Design review of the part built by this model. Coordinates are the model's own, in mm. A direction names the side the tool comes from. Give positions to 0.01 mm unless a question says otherwise; leave off trailing zeros. Order: outer loops, then holes, each group sorted by start corner. A loop starts at its lowest first (then second) coordinate and runs counter-clockwise, first axis right, second up.
```python
from build123d import *

# Parameters (mm, degrees)
F0_W     = 35.8
F0_H     = 9.8
F1_DEPTH = 9.8
F2_R     = 2
F3_DEPTH = 25
F5_DEPTH = 2.4
F6_R     = 2
F7_DEPTH = 40
F8_W     = 2.4
F8_H     = 5.5
F9_DEPTH = 25


with BuildPart() as f1:
    # F0 (on Front) → F1 (new body)
    with BuildSketch(Plane.XZ):
        Rectangle(F0_W, F0_H)
    extrude(amount=F1_DEPTH)

    # F2 (on face) → F3 (cut)
    with BuildSketch(Plane.XZ.offset(9.8)):
        Circle(F2_R)
    extrude(amount=-F3_DEPTH, mode=Mode.SUBTRACT)

    # F4 (on face) → F5 (cut)
    with BuildSketch(Plane.XZ.offset(9.8)):
        Polygon((-1.603947, 2.673454), (-3.117252, -0.052332), (-1.513305, -2.725785), (1.603947, -2.673454), (3.117252, 0.052332), (1.513305, 2.725785), align=None)
    extrude(amount=-F5_DEPTH, mode=Mode.SUBTRACT)

    # F6 (on face) → F7 (cut)
    with BuildSketch(Plane.YZ.offset(17.9)):
        with Locations((-4.9, 0)):
            Circle(F6_R)
    extrude(amount=-F7_DEPTH, mode=Mode.SUBTRACT)

    # F8 (on face) → F9 (cut)
    with BuildSketch(Plane.XZ.offset(9.8)):
        with Locations((6.7, 0)):
            Rectangle(F8_W, F8_H)
        with Locations((-6.7, 0)):
            Rectangle(F8_W, F8_H)
    extrude(amount=-F9_DEPTH, mode=Mode.SUBTRACT)


solid = f1.part
```
1. Take a section at B-B (x = -11). State the section outline as (y, z) points, then the cut area to 3 significant figures.
Recorded:
outline: (-9.8, -4.9) - (0, -4.9) - (0, 4.9) - (-9.8, 4.9) - close; hole circle Ø4 at (-4.9, 0)
area: 83.5 mm2
2. Machinability: for faces 1 (the face through (7, -5, 2.75)), 2 (the face through (3.4, -5.16, 1.983)), 3 (the face through (2, -7.4, 1)), which of the approach directions +Z, -Z, +X, -X, +Y, -Y give a long, thin tool a straight path to every point of the face, cutting with its end or side? Answer none if there is none.
Recorded:
face 1: +Y, -Y
face 2: +X, -X
face 3: -Y
3. For line 1 along X through (y, z) = (-7.25, 2.5); line 2 along Z through (x, y) = (0, -1.6); line 3 along Z through (x, y) = (7, -6.75), list the stretches that pass through material, from the lowest coordinate up.
Recorded:
line 1: x = -17.9 to -7.9, -5.5 to 5.5, 7.9 to 17.9
line 2: z = -4.9 to -2, 2 to 4.9
line 3: z = -4.9 to -2.75, 2.75 to 4.9
4. Draft analysis for pull direction Z (two halves, no side actions). For faces 4 (the face through (5.5, -4, -2)), 5 (the face through (0, -5, -4.9)), 6 (the face through (-0.3, 0, 2.2)), state which applies: pulls with the +Z half, pulls with the -Z half, needs draft (parallel to the pull), parting line crosses it, or undercut.
Recorded:
face 4: undercut
face 5: pulls with the -Z half
face 6: needs draft
5. Take a section at C-C (z = 1.25). State how many separate pieces and enclosed holes the cut face has, then the cut area to 3 significant figures.
Recorded:
separate pieces: 8
enclosed holes: 0
area: 182 mm2
6. Take a section at A-A (y = -1.25). State the section outline as (x, z) points.
Recorded:
outline: (-17.9, -4.9) - (17.9, -4.9) - (17.9, 4.9) - (-17.9, 4.9) - close; hole (-7.9, -2.75) - (-5.5, -2.75) - (-5.5, 2.75) - (-7.9, 2.75) - close; hole circle Ø4 at (0, 0); hole (5.5, -2.75) - (7.9, -2.75) - (7.9, 2.75) - (5.5, 2.75) - close
7. For pin 1 (3 mm diameter, centred on y = -4.9, z = 0, fed in from +X); pin 2 (2.5 mm diameter, centred on x = 0, z = -1, fed in from -Y), all flat-tipped, find the tip position at first contact; note any pin that passes through.
Recorded:
pin 1: passes through
pin 2: stops at y = -7.4
